Can you work these out from the model? Positions are in its coordinate system, mm. Give positions to 0.01 mm unless a question says otherwise; leave off trailing zeros. Order: outer loops, then holes, each group sorted by start corner. A loop starts at its lowest first (then second) coordinate and runs counter-clockwise, first axis right, second up. Notation, with made-up numbers: (63.25, 12) - (86.25, 12) arc R25 ccw to (86.25, 36) - close; hole circle Ø1 at (71, 80). An arc over 180 degrees is marked (long way). Answer as CSV lines item,"result".
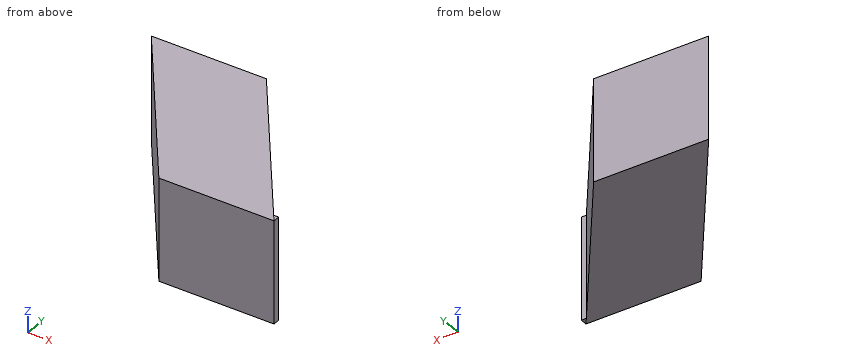
```python
from build123d import *

# Parameters (mm, degrees)
F0_W      = 50.467223
F0_H      = 44.565819
F1_DEPTH  = 3.048
F1_FACE_W = 50.467222
F1_FACE_H = 44.56582


with BuildPart() as f1:
    # F0 (on Front) → F1 (new body)
    with BuildSketch(Plane.XZ):
        with Locations((-0.610485, 7.020649)):
            Rectangle(F0_W, F0_H)
    extrude(amount=F1_DEPTH)

    # F3: sweep along a path in F2
    with BuildLine(Plane.XY) as f3_path:
        Line((-55.554643, 76.514833), (0, 0))
    # F1_face (on face) → F3 (sweep)
    with BuildSketch(Plane(origin=(-0.610486, -3.048, 7.020649), x_dir=(1, 0, 0), z_dir=(0, -1, 0))):
        Rectangle(F1_FACE_W, F1_FACE_H)
    sweep(path=f3_path.line)


solid = f1.part
```
1) I need wall thicknesses on line 1 along Y through (x, z) = (17.5, 10.5); line 2 along X through (y, z) = (18.5, 16); line 3 along Y through (x, z) = (-58, 8). Which ranges of each line are inside material? Lowest first, please. Write a range as [from, to].
Answer block:
line 1,"[-3.05, 6.76]"
line 2,"[-41.49, 8.98]"
line 3,"[41.24, 73.47]"
2) I'm going to push flat-ended pins straight in: P1, Ø6, axis at y = 31, z = 7.5, coming from the -X side; P2, Ø4, axis at x = -66.5, z = 10, coming from the -Y side; P3, Ø2, axis at y = 13.5, z = 16.5, coming from the +X side. Where does each tip first touch, or does it pass through?
Answer block:
P1,"x = -52.74"
P2,"y = 50.19"
P3,"x = 13.33"
3) I want a section at B-B on x = -62. Write out the boundary of the cut face in (y, z).
Answer block:
outline,"(46.75, -15.26) - (73.47, -15.26) - (73.47, 29.3) - (46.75, 29.3) - close"
4) I want a section at A-A on z = -2.5. Write out the boundary of the cut face in (x, y).
Answer block:
outline,"(-81.4, 73.47) - (-25.84, -3.05) - (24.62, -3.05) - (24.62, 0) - (22.41, 0) - (-30.93, 73.47) - close"
5) I want a section at C-C on y = 37.5. Write out the boundary of the cut face in (x, z), plus the area to 3 significant figures.
Answer block:
outline,"(-55.28, -15.26) - (-4.82, -15.26) - (-4.82, 29.3) - (-55.28, 29.3) - close"
area,"2,250 mm2"
